Read the model definition and answer for the solid it produces. Units are mm, in the model's axes. A direction names the side the tool comes from. Coordinates: 2 decimals unless noted, no trailing zeros. Order: outer loops, then holes, each group sorted by start corner. A loop starts at its lowest first (then second) coordinate and runs counter-clockwise, first axis right, second up.
```python
from build123d import *

# Parameters (mm, degrees)
BOSS_EXTRUDE1_DEPTH           = 15
CHAMFER1_SIZE                 = 2.5
SKETCH2_R                     = 1.4
CUT_EXTRUDE1_DEPTH            = 15
CHAMFER2_SIZE                 = 2
SKETCH3_R                     = 1.4
CUT_EXTRUDE2_DEPTH            = 47.129659115
CSK_FOR_M3_SFHCS1_D           = 3
CSK_FOR_M3_SFHCS1_DEPTH       = 31.098709071
CSK_FOR_M3_SFHCS1_CSINK_D     = 6.72
CSK_FOR_M3_SFHCS1_CSINK_ANGLE = 90
CSK_FOR_M3_SFHCS1_TIP         = 0.901290929


with BuildPart() as part:
    # Sketch1 → Boss-Extrude1 (new body)
    with BuildSketch(Plane.XY):
        with BuildLine():
            Line((-19, 0), (-19, -4))
            Line((-19, -4), (-34, -4))
            Line((-34, -4), (-34, 0))
            Line((-34, 0), (-22.883234523, 0))
            ThreePointArc((-22.883234523, 0), (-17.861391251, 14.304304416), (-5, 22.33030278))
            Line((-5, 22.33030278), (-5, 27.33030278))
            Line((-5, 27.33030278), (-1, 27.33030278))
            Line((-1, 27.33030278), (-1, 18.33030278))
            Line((-1, 18.33030278), (-5, 18.33030278))
            ThreePointArc((-5, 18.33030278), (-15.099668871, 11.532562595), (-19, 0))
        make_face()
    extrude(amount=BOSS_EXTRUDE1_DEPTH)

    # Chamfer1
    chamfer1_edges = [part.edges().sort_by_distance(p)[0] for p in [
        (-34, -2, 0),
        (-34, -2, 15),
    ]]
    chamfer(chamfer1_edges, length=CHAMFER1_SIZE)

    # Sketch2 → Cut-Extrude1 (cut)
    with BuildSketch(Plane.ZY.offset(5)):
        with Locations(Location((2.8, 24.83030278, 0), (0, 0, 270))):
            Circle(SKETCH2_R)
        with Locations(Location((12.2, 24.83030278, 0), (0, 0, 270))):
            Circle(SKETCH2_R)
    extrude(amount=-CUT_EXTRUDE1_DEPTH, mode=Mode.SUBTRACT)

    # Chamfer2
    chamfer2_edges = [part.edges().sort_by_distance(p)[0] for p in [
        (-3, 27.33030278, 0),
        (-3, 27.33030278, 15),
    ]]
    chamfer(chamfer2_edges, length=CHAMFER2_SIZE)

    # Sketch3 → Cut-Extrude2 (cut, through all)
    with BuildSketch(Plane(origin=(0, 0, 0), x_dir=(1, 0, 0), z_dir=(0, 1, 0))):
        with Locations(Location((-28.441617262, -7.5, 0), (0, 0, 270))):
            Circle(SKETCH3_R)
    extrude(amount=-CUT_EXTRUDE2_DEPTH, mode=Mode.SUBTRACT)

    # CSK for M3 SFHCS1
    with Locations(Plane(origin=(-28.441617262, 0, 7.5), x_dir=(0, 0, 1), z_dir=(0, 1, 0))):
        with Locations((0, 0)):
            CounterSinkHole(CSK_FOR_M3_SFHCS1_D / 2, CSK_FOR_M3_SFHCS1_CSINK_D / 2, depth=CSK_FOR_M3_SFHCS1_DEPTH, counter_sink_angle=CSK_FOR_M3_SFHCS1_CSINK_ANGLE)
            with Locations((0, 0, -(CSK_FOR_M3_SFHCS1_DEPTH + CSK_FOR_M3_SFHCS1_TIP / 2))):  # 118° drill point
                Cone(0, CSK_FOR_M3_SFHCS1_D / 2, CSK_FOR_M3_SFHCS1_TIP, mode=Mode.SUBTRACT)


solid = part.part
```
1) A cutting plane is placed at A-A, the plane z = 7.5. Determine the outline of the cut face in (x, y).
A:
outline: (-34, -4) - (-29.94, -4) - (-29.94, -1.86) - (-31.8, 0) - (-34, 0) - close; (-26.94, -4) - (-19, -4) - (-19, 0) arc R19 cw to (-5, 18.33) - (-1, 18.33) - (-1, 27.33) - (-5, 27.33) - (-5, 22.33) arc R22.88 ccw to (-22.88, 0) - (-25.08, 0) - (-26.94, -1.86) - close
2) Flat-ended cylindrical pins translate along their axes: pin 1 Ø6 at (y, z) = (5.5, 10.5) entering from -X; pin 2 Ø6 at (y, z) = (8.5, 2) entering from -X; pin 3 Ø4 at (x, z) = (-28.5, 11) entering from +Y; pin 4 Ø1.8 at (x, z) = (-28.44, 7.5) entering from -Y. Find the tip coordinate at first contact, or state that the pin passes through.
A:
pin 1: stops at x = -22.75
pin 2: stops at x = -22.21
pin 3: stops at y = 0
pin 4: passes through
3) A cutting plane is placed at C-C, the plane y = 19.5. Determine the outline of the cut face in (x, z).
A:
outline: (-11.97, 0) - (-1, 0) - (-1, 15) - (-11.97, 15) - close
4) Straight lines are drawn through the part: line 1 (X direction, y = -3, z = 7.5); line 2 (X direction, y = 25, z = 14.25); line 3 (Y direction, x = -28, z = 12.75). For each, find the intervals that lie inside material, in ascending order.
A:
line 1: x = -34 to -29.94, -26.94 to -19
line 2: x = -5 to -1
line 3: y = -4 to 0
5) Which of the six approach directions +Z, -Z, +X, -X, +Y, -Y give full straight-line access (tool end or side, diameter ignored) to faces 1 (the flat face through (-29, 0, 4)), 2 (the flat face through (-32.7, -2, 1.2)), 3 (the flat face through (-19, -2, 7))?
A:
face 1: +Z, -Z, -X, +Y
face 2: -Z, -X, +Y, -Y
face 3: +Z, -Z, +X, -Y
6) A cutting plane is placed at B-B, the plane x = -17.5. Determine the outline of the cut face in (y, z), and give its area (3 significant figures).
A:
outline: (7.4, 0) - (14.74, 0) - (14.74, 15) - (7.4, 15) - close
area: 110 mm2
7) Determine the mould class of faces 4 (the cylindrical face through (-14.994, 11.67, 7.395)), 5 (the cylindrical face through (-29.906, -2.945, 7.825)), 6 (the cylindrical face through (-3.028, 23.495, 3.221)) for opening direction X: pulls with the +X half, pulls with the -X half, needs draft (parallel to the pull), parting line crosses it, or undercut.
A:
face 4: pulls with the +X half
face 5: undercut
face 6: needs draft
